Geometry check sheet. Reference: drawing and pictorial views, mm from the part's lowest x, y, z. A direction names the side the tool comes from. Coordinates: 2 decimals unless noted, no trailing zeros. Loops run counter-clockwise (first coordinate to the right, second up) from the corner with the lowest first, then second, coordinate; pieces in that order, holes last. Notation, with made-up numbers: (-34.5, 36) - (-20.5, 36) arc R22 cw to (-20.5, 62) - close; hole circle Ø3 at (-16, 36.25). An arc over 180 degrees is marked (long way). Write each question's results on one line, items separated by ' | '. Start each with the question number.
1. Cross-section at A-A (x = 6). Record the cut outline in (y, z) (1 decimal).
2. Cross-section at C-C (z = 19). Record the cut outline in (x, y) (1 decimal).
3. Thickness scan on line 1 (Z direction, x = 3.25, y = 156) (1 decimal); line 2 (X direction, y = 270.5, z = 11) (1 decimal). Record the ranges inside material, lowest first. Write a range as [from, to].
4. Gauge pin test, flat ends, axial feed: P1, Ø4, axis at x = 6, z = 10.5, coming from the +Y side; P2, Ø2, axis at y = 87.5, z = 27.5, coming from the +X side (1 decimal). Record the tip position at first contact, or that the pin passes through.
5. Tool access check on the marked faces 1 and 2. Record the directions out of +Z, -Z, +X, -X, +Y, -Y that give a thin tool (end or side, any length) a straight path to the whole face; none if there is none.
6. Cross-section at B-B (y = 162). Record the cut outline in (x, z) (1 decimal).
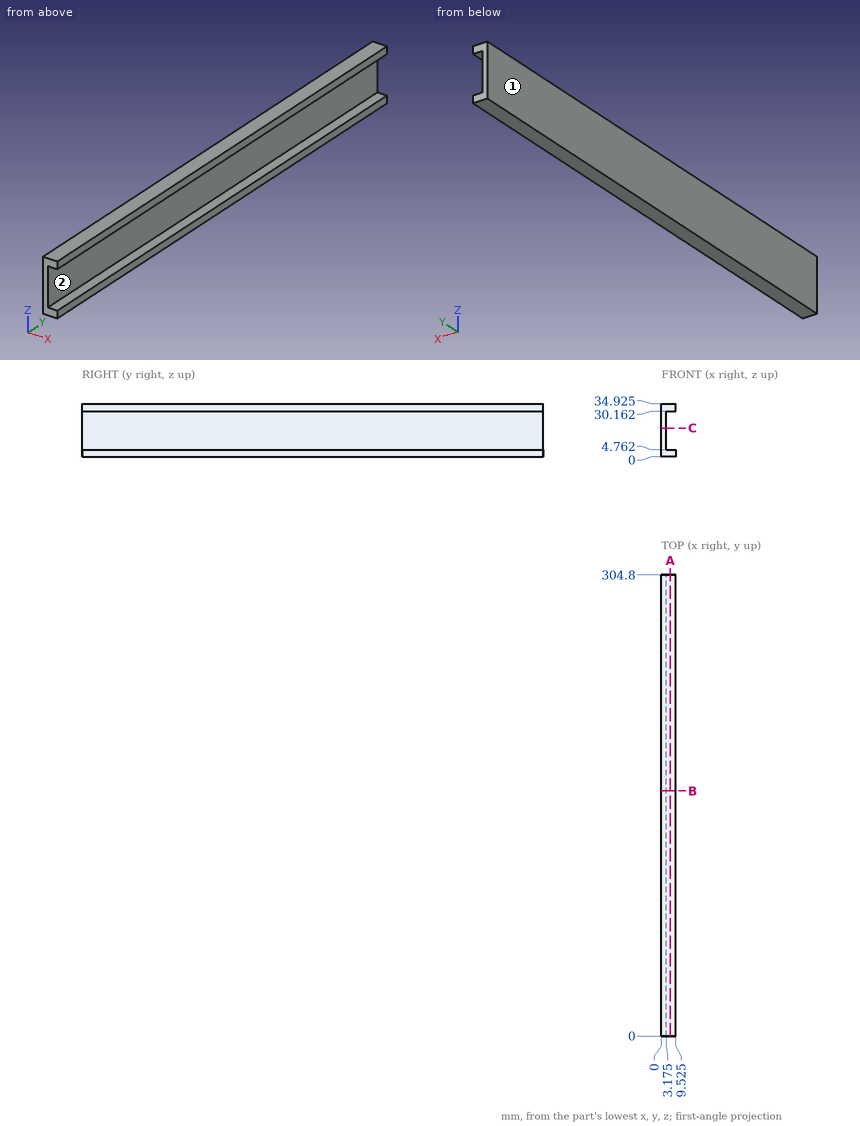
Established:
1) outline: (0, 0) - (304.8, 0) - (304.8, 4.8) - (0, 4.8) - close; (0, 30.2) - (304.8, 30.2) - (304.8, 34.9) - (0, 34.9) - close
2) outline: (0, 0) - (3.2, 0) - (3.2, 304.8) - (0, 304.8) - close
3) line 1: [0, 4.8], [30.2, 34.9] | line 2: [0, 3.2]
4) P1: through | P2: x = 3.2
5) face 1: +Z, -Z, -X, +Y, -Y | face 2: +X, +Y, -Y
6) outline: (0, 0) - (9.5, 0) - (9.5, 4.8) - (3.2, 4.8) - (3.2, 30.2) - (9.5, 30.2) - (9.5, 34.9) - (0, 34.9) - close
